Build history of the part. All positions in model axes, mm. Round coordinates to 2 decimals unless told otherwise and drop trailing zeros. Order: outer loops, then holes, each group sorted by start corner. A loop starts at its lowest first (then second) coordinate and runs counter-clockwise, first axis right, second up. Notation, with made-up numbers: (6.25, 22) -> (43.25, 22) arc R6 ccw to (43.25, 33) -> close; hole circle Ø10 at (59.25, -39.5). An arc over 180 degrees is marked (long way). Write item = value, one per line.
from build123d import *

# Parameters (mm, degrees)
BOSS_EXTRU_1_START = 17.4
ESQUISSE1_R        = 10
BOSS_EXTRU_1_DEPTH = 4


with BuildPart() as part:
    # Esquisse1 → Boss.-Extru.1 (new body)
    with BuildSketch(Plane(origin=(0, 0, 0), x_dir=(1, 0, 0), z_dir=(0, 1, 0)).offset(BOSS_EXTRU_1_START)):
        with Locations(Location((0, 0, 0), (0, 0, 270))):
            Circle(ESQUISSE1_R)
        with BuildLine():
            Line((-1.6, -2.244994432), (-1.6, -2.655183609))
            ThreePointArc((-1.6, -2.655183609), (-0.830340536, -2.986726401), (0, -3.1))
            ThreePointArc((0, -3.1), (3.1, 0), (0, 3.1))
            ThreePointArc((0, 3.1), (-0.830340536, 2.986726401), (-1.6, 2.655183609))
            Line((-1.6, 2.655183609), (-1.6, 2.244994432))
            Line((-1.6, 2.244994432), (-1.6, -2.244994432))
        make_face(mode=Mode.SUBTRACT)
    extrude(amount=BOSS_EXTRU_1_DEPTH)


solid = part.part
Q1. Cut at A-A, the plane z = 0. List the corners of the cut face in (x, y), and give its area (3 significant figures).
Check values:
outline = (-10, 17.4) -> (-1.6, 17.4) -> (-1.6, 21.4) -> (-10, 21.4) -> close; (3.1, 17.4) -> (10, 17.4) -> (10, 21.4) -> (3.1, 21.4) -> close
area = 61.2 mm²
Q2. Cut at C-C, the plane x = 2.5. List the corners of the cut face in (y, z).
Check values:
outline = (17.4, -9.68) -> (21.4, -9.68) -> (21.4, -1.83) -> (17.4, -1.83) -> close; (17.4, 1.83) -> (21.4, 1.83) -> (21.4, 9.68) -> (17.4, 9.68) -> close
Q3. Cut at D-D, the plane x = -7.25. List the corners of the cut face in (y, z).
Check values:
outline = (17.4, -6.89) -> (21.4, -6.89) -> (21.4, 6.89) -> (17.4, 6.89) -> close
Q4. Mould opens along X. For faces 1 (the face through (-9.76, 19.37, -2.17)), 2 (the face through (-2, 17.4, 0)), 3 (the face through (-1.6, 19, 0)) say: released by +X, released by -X, zero draft, split by the parting line, or undercut.
Check values:
face_1 = split by the parting line
face_2 = zero draft
face_3 = undercut
Q5. Flat gauge pins, fed straight in: pin 1 (1 mm diameter, centred on y = 20.5, z = -8, fed in from -X); pin 2 (1.5 mm diameter, centred on y = 18.5, z = 1.5, fed in from -X). Where does each tip first touch, or does it go through?
Check values:
pin_1 = -6.61
pin_2 = -9.97
Q6. Probe probe 1 along Z at (x, y) = (2.5, 19.45); probe 2 along X at (y, z) = (18.6, 2.25); probe 3 along Z at (x, y) = (-1.5, 18.15). List the from-to ranges inside material, lowest first.
Check values:
probe_1 = -9.68 to -1.83, 1.83 to 9.68
probe_2 = -9.74 to -1.6, 2.13 to 9.74
probe_3 = -9.89 to -2.71, 2.71 to 9.89
Q7. Cut at B-B, the plane y = 20.65. List the corners of the cut face in (x, z).
Check values:
outline = circle Ø20 at (0, 0); hole (-1.6, -2.66) arc R3.1 ccw (long way) to (-1.6, 2.66) -> close
